Autodesk Inventor part; units mm, degrees
ref_plane "YZ Plane" through (0, 0, 0) normal (1, 0, 0) x (0, 1, 0)
ref_plane "XZ Plane" through (0, 0, 0) normal (0, 1, 0) x (-1, 0, 0)
ref_plane "XY Plane" through (0, 0, 0) normal (0, 0, 1) x (1, 0, 0)
sketch "Sketch1" plane through (0, 0, 0) normal (0, 0, 1) x (1, 0, 0)
  circle A0 centre (0, 0) radius 11
  circle A1 centre (0, 106.7) radius 11
  line L0 (16, 106.7) -> (16, 53.35)
  line L1 (16, 107.3237) -> (16, 117.7)
  line L2 (16, 117.7) -> (-16, 117.7)
  line L3 (-16, 117.7) -> (-16, 53.35)
  line L4 (11, 0) -> (16, 53.35)
  line L5 (-11, 0) -> (-16, 53.35)
  line L6 (11, 0) -> (16, 53.35)
  line L7 (16, 53.35) -> (16, 117.7)
  line L8 (-16, 117.7) -> (-16, 53.35)
  line L9 (-11, 0) -> (-16, 53.35)
  line L10 (-16, 117.7) -> (16, 117.7)
  line L11 (16, 53.35) -> (-16, 53.35)
  dimension "d1" = 22
  dimension "d2" = 22
  dimension "d3" = 16
  dimension "d4" = 32
extrude "Extrusion1" add sketch "Sketch1" along normal mid plane 48 contours A0 | A0 L5 L11 L4
extrude "Extrusion2" add sketch "Sketch1" along normal mid plane 38 contours A1 | L11 L3 L2 L1 L7 L0
extrude "Extrusion3" add sketch "Sketch1" along normal mid plane 42 contours A1
fillet "Fillet1" radius 2 8 edges at (16, 117.7, 0) (-16, 117.7, 0) (16, 85.525, 19) (-16, 85.525, 19) (-16, 85.525, -19) (16, 85.525, -19) (0, 53.35, -24) (0, 53.35, 24)
sketch "Sketch2" plane through (11, 0, 24) normal (0.9956369, -0.0933118, 0) x (0, 0, -1)
  ellipse E0 centre (2, 51.575) end of major axis (2, 53.5838) minor radius 2 (2, 53.5838) -> (0, 51.575) ccw
  line L0 (48, 0) -> (0, 0)
  line L1 (48, 0) -> (48, 51.575)
  line L2 (0, 0) -> (3, 0)
  line L3 (3, 0) -> (3, 38.5)
  line L4 (3, 38.5) -> (45, 38.5)
  line L5 (45, 38.5) -> (45, -15.2464)
  line L6 (45, -15.2464) -> (3, -15.2464)
  line L7 (3, -15.2464) -> (3, 0)
  point P0 (24, -1.0264)
  dimension "d12" = 3
  dimension "d13" = 38.5
  dimension "d14" = 42
extrude "Extrusion4" cut sketch "Sketch2" along normal mid plane 100
sketch "Sketch3" plane through (0, 0, -24) normal (0, 0, -1) x (-1, 0, 0)
  arc A0 (-11, 0) -> (11, 0) centre (0, 0) ccw
  circle A1 centre (0, 0) radius 5
  dimension "d17" = 10
extrude "Extrusion5" cut sketch "Sketch3" against normal through all
properties part number "Bicep"
Geometry: final body of the model. Coordinates: model frame, mm. A direction names the side the tool comes from. Round coordinates to 2 decimals unless told otherwise and drop trailing zeros. Order: outer loops, then holes, each group sorted by start corner. A loop starts at its lowest first (then second) coordinate and runs counter-clockwise, first axis right, second up.
Q1. Pin query (flat end, axial travel): pin 1 (8.5 mm diameter, centred on x = -6.5, y = 78, fed in from -Z); pin 2 (6 mm diameter, centred on x = 8, y = 96, fed in from -Z); pin 3 (6 mm diameter, centred on x = -5, z = 16.5, fed in from -Y). Return the tip coordinate at first contact, or that it passes through.
Result sheet:
pin 1: stops at z = -19
pin 2: stops at z = -21
pin 3: stops at y = 39.89
Q2. Section C-C, the plane x = -2.5. Give the number of separate pieces and of enclosed holes in the cut face, and give its area (3 significant figures).
Result sheet:
separate pieces: 3
enclosed holes: 0
area: 3,430 mm2
Q3. Section D-D, the plane z = 0.5. Output: boundary loops of the cut face in (x, y).
Result sheet:
outline: (-16, 53.35) - (-14.85, 41.09) - (14.59, 38.33) - (16, 53.35) - (16, 115.7) arc R2 ccw to (14, 117.7) - (-14, 117.7) arc R2 ccw to (-16, 115.7) - close
Q4. Material intervals for probe 1 along Y at (x, z) = (0, 22); probe 2 along Z at (x, y) = (-6.5, 68.5), sorted ascending.
Result sheet:
probe 1: y = -11 to -5, 5 to 53.35
probe 2: z = -19 to 19
Q5. Mould query, pull axis Y, two halves, no side actions, for faces 6 (the face through (-1.432, 95.794, -20.014)), 7 (the face through (0, -11, -23)), 8 (the face through (1, 20, 21)). Classes: released by +Y, released by -Y, zero draft, split by the parting line, or undercut.
Result sheet:
face 6: undercut
face 7: released by -Y
face 8: zero draft
Q6. Section A-A, the plane y = 18. Output: boundary loops of the cut face in (x, z).
Result sheet:
outline: (-12.69, -24) - (12.69, -24) - (12.69, -21) - (-12.69, -21) - close; (-12.69, 21) - (12.69, 21) - (12.69, 24) - (-12.69, 24) - close
Q7. Access query for faces 1 (the face through (0, 107, -21)), 2 (the face through (0, 107, 21)), 3 (the face through (14.785, 40.382, -1.89)), 4 (the face through (-1.432, 95.794, 19.986)), 5 (the face through (-0.34, 39.73, 0.29)). Directions: +Z, -Z, +X, -X, +Y, -Y. A direction counts if a zero-diameter tool reaches every point of the face in a straight line with its end or side. Return the directions, or none.
Result sheet:
face 1: -Z, +X, -X, +Y
face 2: +Z, +X, -X, +Y
face 3: +Z, -Z, +X, -Y
face 4: +Z
face 5: -X, -Y
Q8. Section B-B, the plane y = 81.5. Output: boundary loops of the cut face in (x, z).
Result sheet:
outline: (-16, -17) arc R2 ccw to (-14, -19) - (14, -19) arc R2 ccw to (16, -17) - (16, 17) arc R2 ccw to (14, 19) - (-14, 19) arc R2 ccw to (-16, 17) - close
